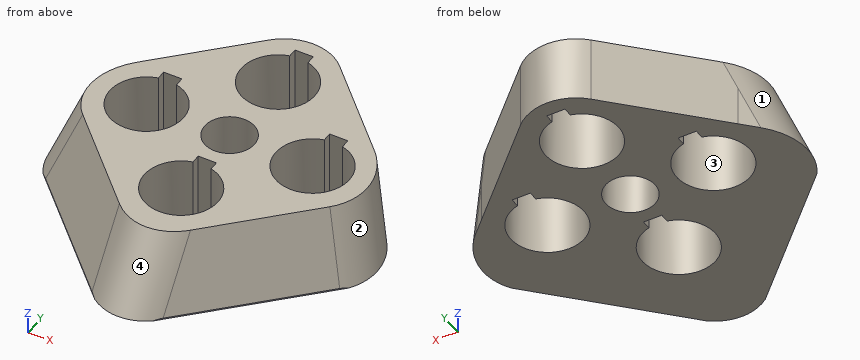
from build123d import *

# Parameters (mm, degrees)
SKETCH1_R           = 7.5
BOSS_EXTRUDE1_DEPTH = 20
FILLET1_R           = 15
BOSS_EXTRUDE2_DEPTH = 20
CHAMFER1_SIZE       = 10
CHAMFER1_SIZE2      = 19.626105055
FILLET2_R           = 17


with BuildPart() as part:
    # Sketch1 → Boss-Extrude1 (new body)
    with BuildSketch(Plane.XY):
        Polygon((0, -24.255339059), (49.255339059, 25), (0, 74.255339059), (-49.255339059, 25), align=None)
        with Locations((0, 25)):
            Circle(SKETCH1_R, mode=Mode.SUBTRACT)
        with BuildLine():
            Line((-2.75, 13.503952762), (2.75, 13.503952762))
            Line((2.75, 13.503952762), (2.75, 10.753952762))
            ThreePointArc((2.75, 10.753952762), (0, -11.1), (-2.75, 10.753952762))
            Line((-2.75, 10.753952762), (-2.75, 13.503952762))
        make_face(mode=Mode.SUBTRACT)
        with BuildLine():
            Line((-2.75, 63.503952762), (2.75, 63.503952762))
            Line((2.75, 63.503952762), (2.75, 60.753952762))
            ThreePointArc((2.75, 60.753952762), (0, 38.9), (-2.75, 60.753952762))
            Line((-2.75, 60.753952762), (-2.75, 63.503952762))
        make_face(mode=Mode.SUBTRACT)
        with BuildLine():
            Line((22.25, 38.503952762), (27.75, 38.503952762))
            Line((27.75, 38.503952762), (27.75, 35.753952762))
            ThreePointArc((27.75, 35.753952762), (25, 13.9), (22.25, 35.753952762))
            Line((22.25, 35.753952762), (22.25, 38.503952762))
        make_face(mode=Mode.SUBTRACT)
        with BuildLine():
            Line((-27.75, 38.503952762), (-22.25, 38.503952762))
            Line((-22.25, 38.503952762), (-22.25, 35.753952762))
            ThreePointArc((-22.25, 35.753952762), (-25, 13.9), (-27.75, 35.753952762))
            Line((-27.75, 35.753952762), (-27.75, 38.503952762))
        make_face(mode=Mode.SUBTRACT)
    extrude(amount=BOSS_EXTRUDE1_DEPTH)

    # Fillet1
    fillet1_edges = [part.edges().sort_by_distance(p)[0] for p in [
        (49.255339059, 25, 10),
        (0, -24.255339059, 10),
        (-49.255339059, 25, 10),
        (0, 74.255339059, 10),
    ]]
    fillet(fillet1_edges, radius=FILLET1_R)

    # Sketch5 → Boss-Extrude2 (add)
    with BuildSketch(Plane(origin=(0, 0, 0), x_dir=(-1, 0, 0), z_dir=(0, 0, -1))):
        Polygon((38.648737342, 35.606601718), (56.326406871, 17.928932188), (0, -38.397474683), (-56.326406871, 17.928932188), (-38.648737342, 35.606601718), (-38.648737342, 14.393398282), (-10.606601718, -13.648737342), (10.606601718, -13.648737342), (38.648737342, 14.393398282), align=None)
    extrude(amount=-BOSS_EXTRUDE2_DEPTH)

    # Chamfer1
    chamfer1_edges = [part.edges().sort_by_distance(p)[0] for p in [
        (-28.163203436, -10.234271247, 20),
        (28.163203436, -10.234271247, 20),
    ]]
    chamfer1_side = [part.faces().sort_by_distance(p)[0] for p in [
        (0, 14.439859593, 20),
    ]]
    chamfer(chamfer1_edges, length=CHAMFER1_SIZE, length2=CHAMFER1_SIZE2, reference=chamfer1_side[0])

    # Fillet2
    # the kernel refuses this fillet: 17 mm, written as the material it takes off along each edge
    with BuildSketch(Plane(origin=(0, -4.097424311, 47.974654117), x_dir=(-0.776565314012209, 0.5111563778483158, -0.3683279387422424), z_dir=(-2.7797289092988672e-15, -0.5846134144132094, -0.8113119965143676))) as fillet2_piece_1:
        with BuildLine():
            CenterArc((FILLET2_R * 0.811311996514, FILLET2_R), FILLET2_R, 191.89433134, 78.10566866)
            Line((-FILLET2_R * 0.167217384978, FILLET2_R * 0.793892626146), (0, 0))
            Line((0, 0), (FILLET2_R * 0.811311996514, 0))
        make_face()
    extrude(amount=93.152096374, mode=Mode.SUBTRACT)
    with BuildSketch(Plane(origin=(35.611999219, 38.643339841, 57.867777278), x_dir=(-0.7071067811865526, -0.7071067811865426, -3.622643282177079e-15), z_dir=(0.3210197609601017, -0.3210197609601017, -0.8910065241883689)), Plane(origin=(-35.611999219, 38.643339841, 57.867777278), x_dir=(0.630036755335051, 0.6300367553350514, -0.45399049973954475), z_dir=(-0.3210197609601016, -0.3210197609601017, -0.8910065241883689))) as fillet2_piece_2:
        with BuildLine():
            CenterArc((FILLET2_R, FILLET2_R), FILLET2_R, 180, 90)
            Line((0, FILLET2_R), (0, 0))
            Line((0, 0), (FILLET2_R, 0))
        make_face()
    extrude(amount=107.026892646, mode=Mode.SUBTRACT)


solid = part.part
Can you work these out from the model? Positions are in its coordinate system, mm. Face numbers are marked on the shaded views. Round coordinates to 2 decimals unless told otherwise and drop trailing zeros. Write each loop counter-clockwise with the first axis right and the second up, starting at its lowest first coordinate (ties: lowest second). Pieces come first, ordered by that corner, then holes. Notation, with made-up numbers: M 57.5,72.5 L 98.5,72.5 A32 cw 98.5,105.5 Z; hole C 32,18.25 d3. An arc over 180 degrees is marked long. Use a Markdown table: item, result.
Item 1: I want a section at B-B (y = 50). List the corners of the cut face in (x, z) for me.
Found:
| item | result |
|---|---|
| outline | M -24.26,0 L -11.1,0 L -11.1,20 L -24.26,20 Z; M 11.1,0 L 24.26,0 L 24.26,20 L 11.1,20 Z |
Item 2: I want a section at D-D (y = 0). List the corners of the cut face in (x, z) for me.
Found:
| item | result |
|---|---|
| outline | M -38.4,0 L -11.1,0 L -11.1,20 L -24.26,20 L -38.4,0.37 Z; M 11.1,0 L 38.4,0 L 38.4,0.37 L 24.26,20 L 11.1,20 Z |
Item 3: If I drill on line 1 along Y through (x, z) = (1.5, 2.5); line 2 along Y through (x, z) = (0, 10.5); line 3 along X through (y, z) = (34, 7), over which ranges is the centre line in solid material (lowest first)? Write a range as [from, to].
Found:
| item | result |
|---|---|
| line 1 | y = [-30.75, -11], [13.5, 17.65], [32.35, 39], [63.5, 67.97] |
| line 2 | y = [-25.07, -11.1], [13.5, 17.5], [32.5, 38.9], [63.5, 68.04] |
| line 3 | x = [-40.26, -31.5], [-18.5, 18.5], [31.5, 40.26] |
Item 4: We'd pull the mould along X, two halves only. Please class the marked faces 1, 2, 3 and 4: released by +X, released by -X, zero draft, split by the parting line, or undercut.
Found:
| item | result |
|---|---|
| face 1 | released by -X |
| face 2 | released by +X |
| face 3 | undercut |
| face 4 | split by the parting line |
Item 5: For pin 1 Ø4 at (y, z) = (49.5, 10) entering from -X; pin 2 Ø6 at (x, z) = (-37.5, 4.5) entering from +Y; pin 3 Ø1.6 at (x, z) = (-0.5, 7) entering from -Y; pin 4 Ø8 at (x, y) = (24.5, -5) entering from +Z, each with a flat end and sliding along its axis, tell me the tip position at first contact or that it passes through.
Found:
| item | result |
|---|---|
| pin 1 | stops at x = -26.76 |
| pin 2 | stops at y = 39.76 |
| pin 3 | stops at y = -28.16 |
| pin 4 | stops at z = 20 |
Item 6: I want a section at A-A (x = 0). List the corners of the cut face in (y, z) for me.
Found:
| item | result |
|---|---|
| outline | M -32.64,0 L -11.1,0 L -11.1,20 L -18.23,20 Z; M 13.5,0 L 17.5,0 L 17.5,20 L 13.5,20 Z; M 32.5,0 L 38.9,0 L 38.9,20 L 32.5,20 Z; M 63.5,0 L 68.04,0 L 68.04,20 L 63.5,20 Z |
Item 7: I want a section at C-C (x = -25.5). List the corners of the cut face in (y, z) for me, and give its area (3 significant figures).
Found:
| item | result |
|---|---|
| outline | M -12.9,0 L 13.91,0 L 13.91,20 L 1.24,20 L -12.9,0.37 Z; M 38.5,0 L 48.76,0 L 48.76,20 L 38.5,20 Z |
| area | 602 mm2 |
